```python
from build123d import *

# Parameters (mm, degrees)
F1_DEPTH = 3.175
F2_T     = -1.5875
F3_R     = 3.175
F4_DEPTH = 2.38125


with BuildPart() as f1:
    # F0 (on Front) → F1 (new body)
    with BuildSketch(Plane.XZ):
        with BuildLine():
            Line((44.45, 0), (-19.05, 0))
            ThreePointArc((-19.05, 0), (-23.540128, -1.859872), (-25.4, -6.35))
            Line((-25.4, -6.35), (-25.4, -76.2))
            ThreePointArc((-25.4, -76.2), (-23.540128, -80.690128), (-19.05, -82.55))
            Line((-19.05, -82.55), (19.05, -82.55))
            Line((19.05, -82.55), (34.108921, -73.855728))
            ThreePointArc((34.108921, -73.855728), (36.696187, -71.024571), (37.181415, -67.220106))
            ThreePointArc((37.181415, -67.220106), (37.699595, -37.354898), (49.657796, -9.983368))
            ThreePointArc((49.657796, -9.983368), (50.080026, -3.413113), (44.45, 0))
        make_face()
    extrude(amount=-F1_DEPTH)

    # F2
    f2_openings = [f1.faces().sort_by_distance(p)[0] for p in [
        (7.276457, 3.175, -39.048077),
    ]]
    offset(amount=F2_T, openings=f2_openings)

    # F3 (on face) → F4 (join)
    with BuildSketch(Plane(origin=(0, 1.5875, 0), x_dir=(-1, 0, 0), z_dir=(0, 1, 0))):
        with Locations((-41.275, -9.525)):
            Circle(F3_R)
        with Locations((-12.7, -9.525)):
            Circle(F3_R)
        with Locations((-30.1625, -34.925)):
            Circle(F3_R)
        with Locations((-22.225, -65.0875)):
            Circle(F3_R)
    extrude(amount=F4_DEPTH)


solid = f1.part
```
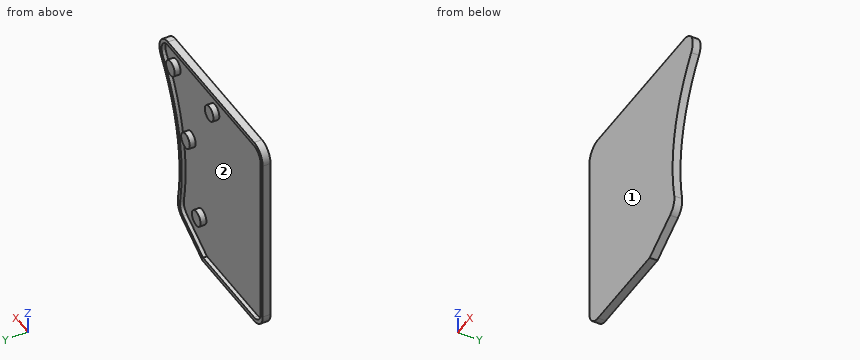
Input: part model. Units: mm. Frame: model coordinates. Face numbers are marked on the shaded views. Give positions to 0.01 mm unless a question says otherwise; leave off trailing zeros. Order: outer loops, then holes, each group sorted by start corner. A loop starts at its lowest first (then second) coordinate and runs counter-clockwise, first axis right, second up. Notation, with made-up numbers: M 17.5,3.5 L 61.5,3.5 A18 ccw 61.5,32.5 Z; hole C -5.75,57 d11. An arc over 180 degrees is marked long. Return JSON: item names as keys, results as strings.
1) Mould query, pull axis X, two halves, no side actions, for the marked faces 1 and 2. Classes: released by +X, released by -X, zero draft, split by the parting line, or undercut.
Taken from the geometry:
{"face 1": "zero draft", "face 2": "undercut"}
2) Section query A-A on y = 2.2. Count the separate pieces of the cut face and the enclosed holes in it, and give its area (3 significant figures).
Taken from the geometry:
{"separate pieces": "5", "enclosed holes": "1", "area": "580 mm2"}
3) Section query C-C on z = -57.5. Output: boundary loops of the cut face in (x, y) (1 decimal), and give its area (3 significant figures).
Taken from the geometry:
{"outline": "M -25.4,0 L 36.1,0 L 36.1,3.2 L 34.5,3.2 L 34.5,1.6 L -23.8,1.6 L -23.8,3.2 L -25.4,3.2 Z", "area": "103 mm2"}
4) Line query: L1, parallel to Z at x = 2.5, y = 3; L2, parallel to X at y = 2.4, z = -10; L3, parallel to Y at x = 8, z = -49.5. Output: solid intervals per line, ascending. Write a range as [from, to].
Taken from the geometry:
{"L1": "z = [-82.55, -80.96], [-1.59, 0]", "L2": "x = [-25.4, -23.81], [9.56, 15.84], [38.14, 44.41], [47.72, 49.65]", "L3": "y = [0, 1.59]"}
5) Contact query for flat-ended pins moving along their axis: pin 1 (6 mm diameter, centred on x = 14, z = -48, fed in from +Y); pin 2 (0.8 mm diameter, centred on x = 23, y = 2, fed in from -Z); pin 3 (0.8 mm diameter, centred on y = 2.5, z = -26, fed in from +X). Output: stop coordinate, or through.
Taken from the geometry:
{"pin 1": "stops at y = 1.59", "pin 2": "stops at z = -80.5", "pin 3": "stops at x = 41.28"}
